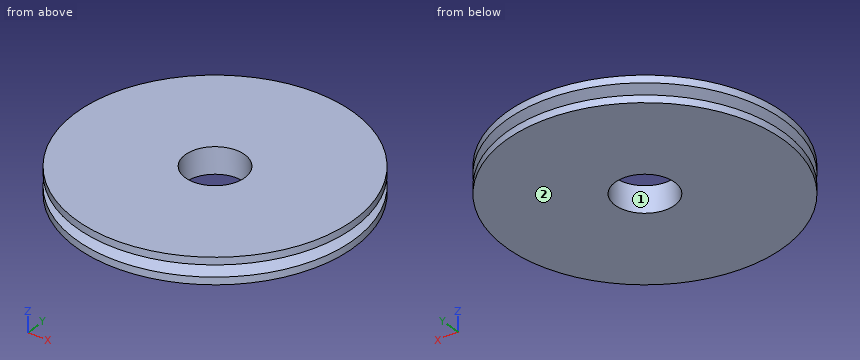
Autodesk Inventor part; units mm, degrees
ref_plane "Plan de courroie" through (0, 105.5, 11) normal (0, 0, 1) x (1, 0, 0)
ref_plane "YZ Plane" through (0, 0, 0) normal (1, 0, 0) x (0, 1, 0)
ref_plane "XZ Plane" through (0, 0, 0) normal (0, 1, 0) x (-1, 0, 0)
sketch "Esquisse principale" plane through (0, 0, 0) normal (1, 0, 0) x (0, 1, 0)
  line L0 (0, 22) -> (116.5, 22)
  line L1 (116.5, 22) -> (116.5, 15.8615)
  line L2 (116.5, 15.8615) -> (105.5, 12.4984)
  line L3 (105.5, 12.4984) -> (105.5, 9.5016)
  line L4 (105.5, 9.5016) -> (116.5, 6.1385)
  line L5 (116.5, 6.1385) -> (116.5, 0)
  line L6 (116.5, 0) -> (0, 0)
  line L7 (114.5, 15.25) -> (114.5, 6.75) construction
  line L8 (105.5, 11) -> (114.5, 11) construction
  line L9 (116.5, 15.8615) -> (116.5, 6.1385)
  line L10 (0, -3.2) -> (0, 19.2)
  line L11 (0, 0) -> (0, 22)
  dimension "d0" = 8.5
  dimension "d1" = 34
  dimension "d2" = 2
  dimension "d6" = 22
  dimension "d21" = 229
  dimension "d25" = 11
  dimension "d27" = 11
ref_plane "Plan de courroie" through (0, 105.5, 11) normal (0, 0, 1) x (1, 0, 0)
revolve "Corps" add sketch "Esquisse principale" angle 360 about axis through (0, 0, -10) along (0, 0, 1)
revolve "Bord" cut sketch "Esquisse principale" angle 360 about axis through (0, 0, -10) along (0, 0, 1) contours L9 L4 L3 L2
fillet "Congé externe" [suppressed]
fillet "Congé interne" [suppressed]
pattern_of_one "Réseau de bords"
sketch "Esquisse2" plane through (0, 0, 22) normal (0, 0, 1) x (1, 0, 0)
  circle A0 centre (0, 0) radius 116.5
hole "Perçage1" at (0, 0, 22) direction (0, 0, -1) diameter 50 depth 22
equation "\"d0\" = da_Bw"
equation "\"d1\" = da_Alfa"
equation "\"d2\" = da_c"
equation "\"d21\" = da_Dw"
equation "\"d25\" = da_Hd"
equation "\"d27\" = da_Se"
equation "\"da_r1\" = 0"
equation "\"da_r2\" = 0"
equation "\"d18\" = da_Sg"
equation "\"d5\" = da_Se"
equation "\"da_Bw\" = 8.5"
equation "\"da_Alfa\" = 34deg"
equation "\"da_c\" = 2"
equation "\"da_Dw\" = 229"
equation "\"da_Hd\" = 11"
equation "\"da_Se\" = 11"
equation "\"da_Sg\" = 12"
properties part number "Poulie à gorge1" material "Steel"
Build history of the part. All positions in model axes, mm. Face numbers are marked on the shaded views. Coordinates: 2 decimals unless noted, no trailing zeros. Order: outer loops, then holes, each group sorted by start corner. A loop starts at its lowest first (then second) coordinate and runs counter-clockwise, first axis right, second up. Notation, with made-up numbers: (82, 42) -> (127, 42) arc R14 ccw to (127, 63) -> close; hole circle Ø6 at (-20.5, 48.5). An arc over 180 degrees is marked (long way). One line per item, written item: value.
(1) Slice it at C-C, the plane z = 2.75. List the corners of the cut face in (x, y), plus the area to 3 significant figures.
Checked values:
outline: circle Ø233 at (0, 0); hole circle Ø50 at (0, 0)
area: 40,700 mm2
(2) Mould opens along X. For the marked faces 1 and 2 say: pulls with the +X half, pulls with the -X half, needs draft (parallel to the pull), parting line crosses it, or undercut.
Checked values:
face 1: undercut
face 2: needs draft
(3) Slice it at A-A, the plane x = 0. List the corners of the cut face in (y, z), plus the area to 3 significant figures.
Checked values:
outline: (-116.5, 0) -> (-25, 0) -> (-25, 22) -> (-116.5, 22) -> (-116.5, 15.86) -> (-105.5, 12.5) -> (-105.5, 9.5) -> (-116.5, 6.14) -> close; (25, 0) -> (116.5, 0) -> (116.5, 6.14) -> (105.5, 9.5) -> (105.5, 12.5) -> (116.5, 15.86) -> (116.5, 22) -> (25, 22) -> close
area: 3,890 mm2
(4) Probe line 1 (X direction, y = 0, z = 6); line 2 (Y direction, x = 19, z = 1). List the from-to ranges inside material, lowest first. Write a range as [from, to].
Checked values:
line 1: [-116.5, -25], [25, 116.5]
line 2: [-114.94, -16.25], [16.25, 114.94]
(5) Drop flat-ended pins along their axis: pin 1 Ø1 at (y, z) = (23.5, 18.5) entering from -X; pin 2 Ø10 at (x, z) = (41.5, 6) entering from -Y; pin 3 Ø2 at (y, z) = (-62, 5.5) entering from -X. Give the stop position or say it passes through.
Checked values:
pin 1: x = -114.21
pin 2: y = -110.63
pin 3: x = -99.25
